Here's how the part is built. I have some questions about the finished solid (model axes, mm). Round coordinates to 2 decimals unless told otherwise and drop trailing zeros. Order: outer loops, then holes, each group sorted by start corner. A loop starts at its lowest first (then second) coordinate and runs counter-clockwise, first axis right, second up. Notation, with made-up numbers: (-27, -13) - (-1, -13) arc R28 ccw to (-1, 14) - close; hole circle Ø1 at (76.25, 85). An arc over 180 degrees is marked (long way). One line per item, written item: value.
Autodesk Inventor part; units mm, degrees
ref_plane "YZ Plane" through (0, 0, 0) normal (1, 0, 0) x (0, 1, 0)
ref_plane "XZ Plane" through (0, 0, 0) normal (0, 1, 0) x (-1, 0, 0)
ref_plane "XY Plane" through (0, 0, 0) normal (0, 0, 1) x (1, 0, 0)
sketch "Sketch1" plane through (0, 0, 0) normal (0, 1, 0) x (-1, 0, 0)
  line L0 (95, -95) -> (-95, -95)
  line L1 (-95, -95) -> (-95, 95)
  line L2 (-95, 95) -> (95, 95)
  line L3 (95, 95) -> (95, -95)
  line L4 (95, -95) -> (-95, 95) construction
  line L5 (-95, -95) -> (95, 95) construction
  point P0 (0, 0)
  dimension "d0" = 190
extrude "Extrusion1" add sketch "Sketch1" along normal blind 1.5875
sketch "Sketch2" plane through (0, 1.5875, 0) normal (0, 1, 0) x (1, 0, 0)
  line L0 (-95, 95) -> (-95, -95)
  line L1 (-95, -95) -> (95, -95)
  line L2 (95, 95) -> (-95, 95)
  line L3 (-95, 95) -> (-95, -95)
  line L4 (-95, -95) -> (95, -95)
  line L5 (95, -95) -> (95, 95)
  point P0 (-85, 0)
  point P1 (0, -85)
  point P2 (85, 0)
  point P3 (0, 85)
  point P4 (0, 0)
  dimension "d17" = 10
  dimension "d18" = 10
  dimension "d19" = 10
  dimension "d20" = 10
hole "Hole1" at (-85, 1.5875, 0) at (0, 1.5875, 85) at (85, 1.5875, 0) at (0, 1.5875, -85) direction (0, -1, 0) diameter 5.5 end through all
properties part number "short covering" material "Glass"
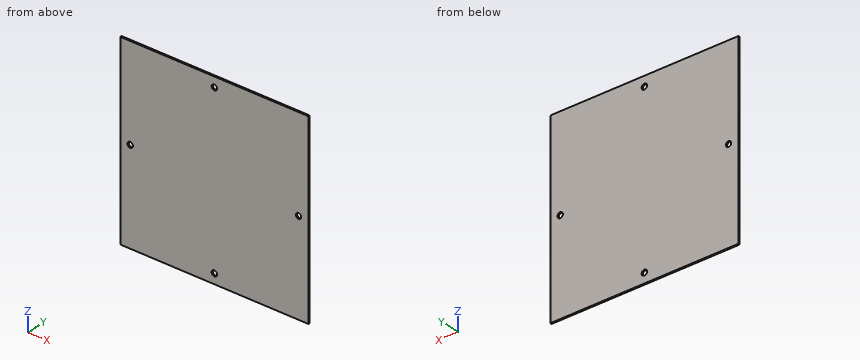
Q1. If we section it at C-C, the plane x = 85: Please give me the cut outline in (y, z), then the cut area to 3 significant figures.
Results list:
outline: (0, -95) - (1.59, -95) - (1.59, -2.75) - (0, -2.75) - close; (0, 2.75) - (1.59, 2.75) - (1.59, 95) - (0, 95) - close
area: 293 mm²
Q2. If I drill on line 1 along Z through (x, y) = (0, 0.9); line 2 along Z through (x, y) = (-85, 0.75), over which ranges is the centre line in solid material (lowest first)?
Results list:
line 1: -95 to -87.75, -82.25 to 82.25, 87.75 to 95
line 2: -95 to -2.75, 2.75 to 95
Q3. If we section it at D-D, the plane z = 0: Please give me the cut outline in (x, y).
Results list:
outline: (-95, 0) - (-87.75, 0) - (-87.75, 1.59) - (-95, 1.59) - close; (-82.25, 0) - (82.25, 0) - (82.25, 1.59) - (-82.25, 1.59) - close; (87.75, 0) - (95, 0) - (95, 1.59) - (87.75, 1.59) - close
Q4. If we section it at B-B, the plane x = 0: Please give me the cut outline in (y, z).
Results list:
outline: (0, -95) - (1.59, -95) - (1.59, -87.75) - (0, -87.75) - close; (0, -82.25) - (1.59, -82.25) - (1.59, 82.25) - (0, 82.25) - close; (0, 87.75) - (1.59, 87.75) - (1.59, 95) - (0, 95) - close
Q5. If we section it at A-A, the plane z = 85: Please give me the cut outline in (x, y), then the cut area to 3 significant figures.
Results list:
outline: (-95, 0) - (-2.75, 0) - (-2.75, 1.59) - (-95, 1.59) - close; (2.75, 0) - (95, 0) - (95, 1.59) - (2.75, 1.59) - close
area: 293 mm²
Q6. Will this pin go through, and if not, where does the flat tip stop? pin 1 (4.5 mm diameter, centred on x = -85, z = 0, fed in from +Y).
Results list:
pin 1: through
